Design review of the part built by this model. Coordinates are the model's own, in mm. A direction names the side the tool comes from. Round coordinates to 2 decimals unless told otherwise and drop trailing zeros. Write each loop counter-clockwise with the first axis right and the second up, starting at its lowest first coordinate (ties: lowest second). Pieces come first, ordered by that corner, then holes. Notation, with made-up numbers: (88, -36.75) -> (141, -36.75) arc R37 cw to (141, -0.75) -> close; hole circle Ø10 at (20.25, -26). An arc over 180 degrees is marked (long way). Write item = value, one per line. Start each with the question number.
Item 1: For pin 1 Ø6 at (x, z) = (63.5, -57) entering from -Y; pin 2 Ø0.9 at (x, y) = (5, 4.5) entering from -Z; pin 3 Ø3 at (y, z) = (4, -61) entering from +X; pin 4 Ø1 at (y, z) = (5.5, -50.5) entering from -X, all flat-tipped, find the tip position at first contact; note any pin that passes through.
Item 2: Machinability: for faces 1 (the cylindrical face through (17.45, 3.22, -31.18)), 2 (the flat face through (7, 3, -63)), 3 (the flat face through (56, 3, -56.5)), 4 (the flat face through (38, 3, -27.1)), which of the approach directions +Z, -Z, +X, -X, +Y, -Y give a long, thin tool a straight path to every point of the face, cutting with its end or side? Answer none if there is none.
Item 3: Add section D-D, the plane z = -64. State the section outline as (x, y) points.
Item 4: Add section A-A, the plane x = 12.5. State the section outline as (y, z) points, then the cut area to 3 significant figures.
Item 5: Add section C-C, the plane y = 4.5. State the section outline as (x, z) points.
Item 6: To check wall thickness, follow L1, parallel to X at y = 1.5, z = -61.75; L2, parallel to X at y = 2.75, z = -40; L3, parallel to Z at x = 23, y = 3.5. State the ranges of each line that lie inside material, in increasing order.
Item 7: Add section B-B, the plane z = -36. State the section outline as (x, y) points, then the cut area to 3 significant figures.
Item 8: Mouldability with a two-part tool opening along X and no side actions: class faces 5 (the cylindrical face through (33.55, 3.22, -67.07)), 6 (the flat face through (3.545, 3.131, -53.565)), 7 (the cylindrical face through (7.5, 3.1, -47.3)) as released by +X, released by -X, zero draft, split by the parting line, or undercut.
from build123d import *

# Parameters (mm, degrees)
SKETCH1_R           = 2
SKETCH1_R_2         = 3
SKETCH1_W           = 13
SKETCH1_H           = 8.25
BOSS_EXTRUDE1_DEPTH = 6.35
FILLET1_R           = 1.5
SKETCH2_W           = 82.327825706
SKETCH2_H           = 14.458254131
CUT_EXTRUDE1_DEPTH  = 51
SKETCH3_W           = 51.5
SKETCH3_H           = 6.35
BOSS_EXTRUDE2_DEPTH = 25
SKETCH4_W           = 84.929028447
SKETCH4_H           = 25.885902506
CUT_EXTRUDE2_DEPTH  = 90
SKETCH5_W           = 0.1
SKETCH5_H           = 6.35
CUT_EXTRUDE3_DEPTH  = 90
SKETCH6_W           = 81.24526446
SKETCH6_H           = 21.013173112
CUT_EXTRUDE4_DEPTH  = 90


with BuildPart() as part:
    # Sketch1 → Boss-Extrude1 (new body)
    with BuildSketch(Plane(origin=(0, 0, 0), x_dir=(1, 0, 0), z_dir=(0, 1, 0))):
        Polygon((38, 0), (38, 5), (58, 5), (58, 0), (96, 0), (96, 48.5), (89, 58.5), (89, 67.5), (62, 67.5), (62, 56.5), (34, 56.5), (34, 67.5), (7, 67.5), (7, 58.5), (0, 48.5), (0, 0), align=None)
        with Locations(Location((38.5, 40, 0), (0, 0, 270))):
            Circle(SKETCH1_R, mode=Mode.SUBTRACT)
        with Locations(Location((38.5, 22, 0), (0, 0, 270))):
            Circle(SKETCH1_R, mode=Mode.SUBTRACT)
        with Locations(Location((57.5, 22, 0), (0, 0, 90))):
            Circle(SKETCH1_R, mode=Mode.SUBTRACT)
        with Locations(Location((57.5, 40, 0), (0, 0, 90))):
            Circle(SKETCH1_R, mode=Mode.SUBTRACT)
        with Locations(Location((12.5, 61.75, 0), (0, 0, 270))):
            Circle(SKETCH1_R_2, mode=Mode.SUBTRACT)
        with Locations(Location((28, 61.75, 0), (0, 0, 270))):
            Circle(SKETCH1_R_2, mode=Mode.SUBTRACT)
        with Locations(Location((68, 61.75, 0), (0, 0, 90))):
            Circle(SKETCH1_R_2, mode=Mode.SUBTRACT)
        with Locations(Location((83.5, 61.75, 0), (0, 0, 90))):
            Circle(SKETCH1_R_2, mode=Mode.SUBTRACT)
        with Locations((72.5, 18.625)):
            Rectangle(SKETCH1_W, SKETCH1_H, mode=Mode.SUBTRACT)
        with Locations((23.5, 34.875)):
            Rectangle(SKETCH1_W, SKETCH1_H, mode=Mode.SUBTRACT)
        with Locations((23.5, 18.625)):
            Rectangle(SKETCH1_W, SKETCH1_H, mode=Mode.SUBTRACT)
        with Locations((72.5, 34.875)):
            Rectangle(SKETCH1_W, SKETCH1_H, mode=Mode.SUBTRACT)
        with BuildLine():
            Line((2.75, 11.75), (5.75, 11.75))
            ThreePointArc((5.75, 11.75), (7.5, 10), (5.75, 8.25))
            Line((5.75, 8.25), (2.75, 8.25))
            ThreePointArc((2.75, 8.25), (1, 10), (2.75, 11.75))
        make_face(mode=Mode.SUBTRACT)
        with BuildLine():
            Line((93.25, 8.25), (90.25, 8.25))
            ThreePointArc((90.25, 8.25), (88.5, 10), (90.25, 11.75))
            Line((90.25, 11.75), (93.25, 11.75))
            ThreePointArc((93.25, 11.75), (95, 10), (93.25, 8.25))
        make_face(mode=Mode.SUBTRACT)
        with BuildLine():
            Line((93.25, 45.5), (90.25, 45.5))
            ThreePointArc((90.25, 45.5), (88.5, 47.25), (90.25, 49))
            Line((90.25, 49), (93.25, 49))
            ThreePointArc((93.25, 49), (95, 47.25), (93.25, 45.5))
        make_face(mode=Mode.SUBTRACT)
        with BuildLine():
            Line((2.75, 49), (5.75, 49))
            ThreePointArc((5.75, 49), (7.5, 47.25), (5.75, 45.5))
            Line((5.75, 45.5), (2.75, 45.5))
            ThreePointArc((2.75, 45.5), (1, 47.25), (2.75, 49))
        make_face(mode=Mode.SUBTRACT)
    extrude(amount=BOSS_EXTRUDE1_DEPTH)

    # Fillet1
    fillet1_edges = [part.edges().sort_by_distance(p)[0] for p in [
        (0, 3.175, -48.5),
        (7, 3.175, -58.5),
        (7, 3.175, -67.5),
        (34, 3.175, -67.5),
        (34, 3.175, -56.5),
        (62, 3.175, -56.5),
        (62, 3.175, -67.5),
        (89, 3.175, -67.5),
        (89, 3.175, -58.5),
        (96, 3.175, -48.5),
        (96, 3.175, 0),
        (58, 3.175, 0),
        (58, 3.175, -5),
        (38, 3.175, -5),
        (38, 3.175, 0),
        (0, 3.175, 0),
        (17, 3.175, -39),
        (17, 3.175, -30.75),
        (30, 3.175, -30.75),
        (30, 3.175, -39),
        (17, 3.175, -22.75),
        (17, 3.175, -14.5),
        (30, 3.175, -14.5),
        (30, 3.175, -22.75),
        (79, 3.175, -14.5),
        (79, 3.175, -22.75),
        (66, 3.175, -22.75),
        (66, 3.175, -14.5),
        (79, 3.175, -30.75),
        (79, 3.175, -39),
        (66, 3.175, -39),
        (66, 3.175, -30.75),
    ]]
    fillet(fillet1_edges, radius=FILLET1_R)

    # Sketch2 → Cut-Extrude1 (cut)
    with BuildSketch(Plane(origin=(48, 0, 0), x_dir=(0, 0, -1), z_dir=(1, 0, 0))):
        with Locations((33.293792952, 1.315835649)):
            Rectangle(SKETCH2_W, SKETCH2_H)
    extrude(amount=CUT_EXTRUDE1_DEPTH, mode=Mode.SUBTRACT)

    # Sketch3 → Boss-Extrude2 (add)
    with BuildSketch(Plane(origin=(48, 0, 0), x_dir=(0, 0, -1), z_dir=(1, 0, 0))):
        with Locations((30.75, 3.175)):
            Rectangle(SKETCH3_W, SKETCH3_H)
    extrude(amount=BOSS_EXTRUDE2_DEPTH)

    # Mirror1: part across plane


with BuildPart() as part_1:
    add(part.part)
    add(part.part.mirror(Plane(origin=(73, 0, 0), x_dir=(0, 0, 1), z_dir=(1, 0, 0))))

    # Sketch4 → Cut-Extrude2 (cut)
    with BuildSketch(Plane(origin=(75, 0, 0), x_dir=(0, 0, -1), z_dir=(1, 0, 0))):
        with Locations((34.029781947, 1.13903014)):
            Rectangle(SKETCH4_W, SKETCH4_H)
    extrude(amount=CUT_EXTRUDE2_DEPTH, mode=Mode.SUBTRACT)

    # Sketch5 → Cut-Extrude3 (cut)
    with BuildSketch(Plane(origin=(75, 0, 0), x_dir=(0, 0, -1), z_dir=(1, 0, 0))):
        with Locations((27.05, 3.175)):
            Rectangle(SKETCH5_W, SKETCH5_H)
    extrude(amount=-CUT_EXTRUDE3_DEPTH, mode=Mode.SUBTRACT)


with BuildPart() as cut_extrude3_piece_1:
    # of the separate pieces the step leaves, piece 1, a body of its own (cut_extrude3_pieces)
    add(part_1.part.solids().sort_by_distance((0, 0, -48.027166654))[0])


with BuildPart() as cut_extrude3_piece_2:
    # of the separate pieces the step leaves, piece 2, a body of its own (cut_extrude3_pieces)
    add(part_1.part.solids().sort_by_distance((38, 0, -1.5))[0])

    # Sketch6 → Cut-Extrude4 (cut)
    with BuildSketch(Plane(origin=(0, 0, -27), x_dir=(-1, 0, 0), z_dir=(0, 0, -1))):
        with Locations((-35.926138856, 1.728749219)):
            Rectangle(SKETCH6_W, SKETCH6_H)
    extrude(amount=-CUT_EXTRUDE4_DEPTH, mode=Mode.SUBTRACT)


solid = cut_extrude3_piece_1.part
Result set:
q1.pin_1 = 0
q1.pin_2 = -56.29
q1.pin_3 = 34
q1.pin_4 = 1.05
q2.face_1 = +Y, -Y
q2.face_2 = -Z, -X, +Y, -Y
q2.face_3 = -Z, +X, +Y, -Y
q2.face_4 = +Z, +X, -X, +Y, -Y
q3.outline = (7, 0) -> (10.52, 0) -> (10.52, 6.35) -> (7, 6.35) -> close; (14.48, 0) -> (26.02, 0) -> (26.02, 6.35) -> (14.48, 6.35) -> close; (29.98, 0) -> (34, 0) -> (34, 6.35) -> (29.98, 6.35) -> close
q4.outline = (0, -67.5) -> (6.35, -67.5) -> (6.35, -64.75) -> (0, -64.75) -> close; (0, -58.75) -> (6.35, -58.75) -> (6.35, -27.1) -> (0, -27.1) -> close
q4.area = 218 mm²
q5.outline = (0, -48.03) arc R1.5 ccw to (0.27, -48.89) -> (6.73, -58.11) arc R1.5 cw to (7, -58.97) -> (7, -66) arc R1.5 ccw to (8.5, -67.5) -> (32.5, -67.5) arc R1.5 ccw to (34, -66) -> (34, -58) arc R1.5 cw to (35.5, -56.5) -> (75, -56.5) -> (75, -27.1) -> (0, -27.1) -> close; hole (2.75, -49) -> (5.75, -49) arc R1.75 ccw to (5.75, -45.5) -> (2.75, -45.5) arc R1.75 ccw to start; hole circle Ø6 at (12.5, -61.75); hole (17, -37.5) arc R1.5 ccw to (18.5, -39) -> (28.5, -39) arc R1.5 ccw to (30, -37.5) -> (30, -32.25) arc R1.5 ccw to (28.5, -30.75) -> (18.5, -30.75) arc R1.5 ccw to (17, -32.25) -> close; hole circle Ø6 at (28, -61.75); hole circle Ø4 at (38.5, -40)
q6.L1 = 7 to 9.5, 15.5 to 25, 31 to 34
q6.L2 = 0 to 36.5, 40.5 to 75
q6.L3 = -67.5 to -39, -30.75 to -27.1
q7.outline = (0, 0) -> (17, 0) -> (17, 6.35) -> (0, 6.35) -> close; (30, 0) -> (75, 0) -> (75, 6.35) -> (30, 6.35) -> close
q7.area = 394 mm²
q8.face_5 = released by +X
q8.face_6 = released by -X
q8.face_7 = undercut
